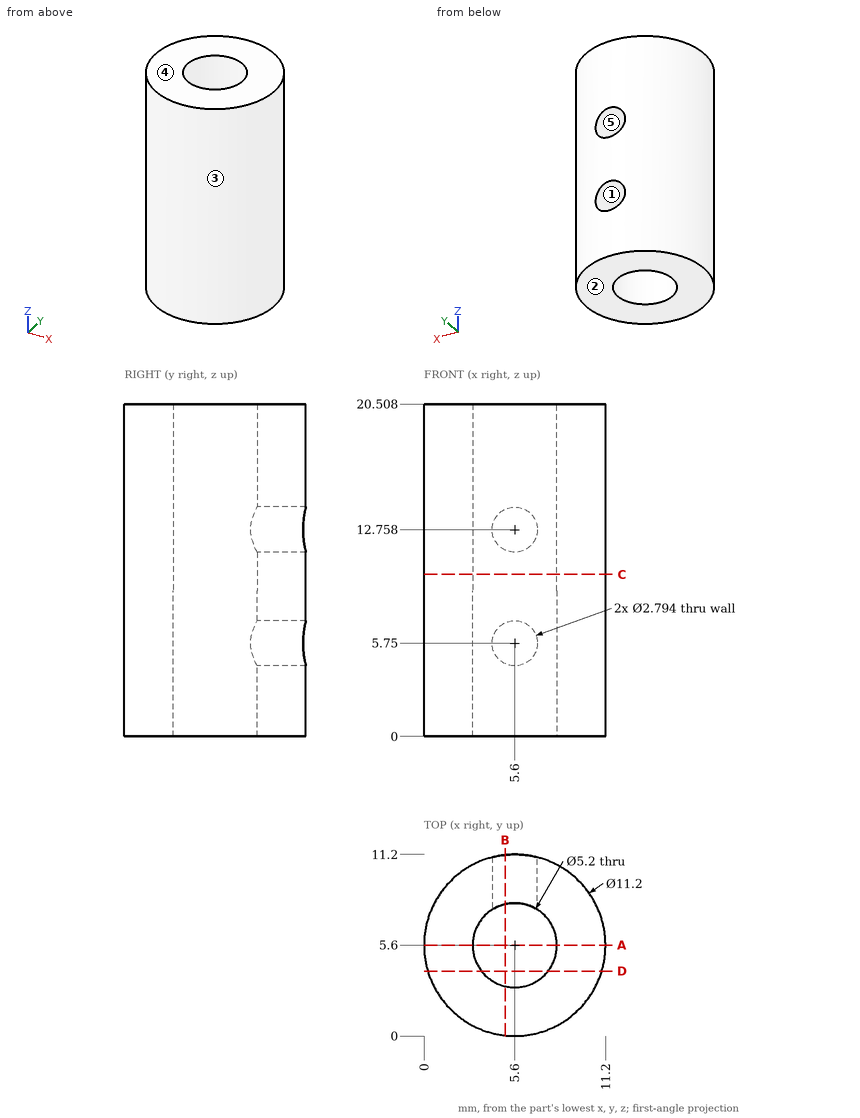
Geometry: see drawing. Coordinates: mm, zero at the bounding-box minimum. A direction names the side the tool comes from. Coordinates: 2 decimals unless noted, no trailing zeros. Write each loop counter-clockwise with the first axis right and the second up, starting at its lowest first coordinate (ties: lowest second). Pieces come first, ordered by that corner, then holes. Notation, with made-up numbers: M 6.25,24.5 L 34.25,24.5 A29 cw 34.25,61.5 Z; hole C -31.75,54.25 d7. An arc over 180 degrees is marked long. Use CSV: the item, a comma, the result in double quotes. Start each with the question number.
1. Ray query, probe 1 along Z at (x, y) = (5.6, 8.95) (3 decimals); probe 2 along Y at (x, z) = (5.6, 3). Return the intervals inside material, ascending.
2. Cut plane C-C on z = 10. Return the cut outline in (x, y).
3. Mould query, pull axis X, two halves, no side actions, for the marked faces 1, 2 and 3. Classes: pulls with the +X half, pulls with the -X half, needs draft (parallel to the pull), parting line crosses it, or undercut.
4. Reachability of the marked faces 4 and 5 from +Z, -Z, +X, -X, +Y, -Y: full face, straight path, thin tool, end or side. Return the list, or none.
5. Cut plane D-D on y = 4. Return the cut outline in (x, z).
6. First-contact query: P1, Ø6, axis at x = 9.5, z = 18.5, coming from the +Y side; P2, Ø2.5, axis at x = 5.6, z = 12.758, coming from the +Y side; P3, Ø3, axis at x = 7.5, z = 9.5, coming from the +Y side. Flat tips, straight axial feed; report the tip coordinate or a pass-through.
7. Cut plane A-A on y = 5.6. Return the cut outline in (x, z), plus the area to 3 significant figures.
8. Cut plane B-B on x = 5. Return the cut outline in (y, z).
Entries:
1,probe 1,"0 to 4.353, 7.147 to 11.361, 14.155 to 20.508"
1,probe 2,"0 to 3, 8.2 to 11.2"
2,outline,"C 5.6,5.6 d11.2; hole C 5.6,5.6 d5.2"
3,face 1,"undercut"
3,face 2,"needs draft"
3,face 3,"parting line crosses it"
4,face 4,"+Z, +X, -X, +Y, -Y"
4,face 5,"+Y"
5,outline,"M 0.23,0 L 3.55,0 L 3.55,20.51 L 0.23,20.51 Z; M 7.65,0 L 10.97,0 L 10.97,20.51 L 7.65,20.51 Z"
6,P1,"y = 11.13"
6,P2,"y = 3.32"
6,P3,"y = 11.19"
7,outline,"M 0,0 L 3,0 L 3,20.51 L 0,20.51 Z; M 8.2,0 L 11.2,0 L 11.2,20.51 L 8.2,20.51 Z"
7,area,"123 mm²"
8,outline,"M 0.03,0 L 3.07,0 L 3.07,20.51 L 0.03,20.51 Z; M 8.13,0 L 11.17,0 L 11.17,4.49 L 8.13,4.49 Z; M 8.13,7.01 L 11.17,7.01 L 11.17,11.5 L 8.13,11.5 Z; M 8.13,14.02 L 11.17,14.02 L 11.17,20.51 L 8.13,20.51 Z"
